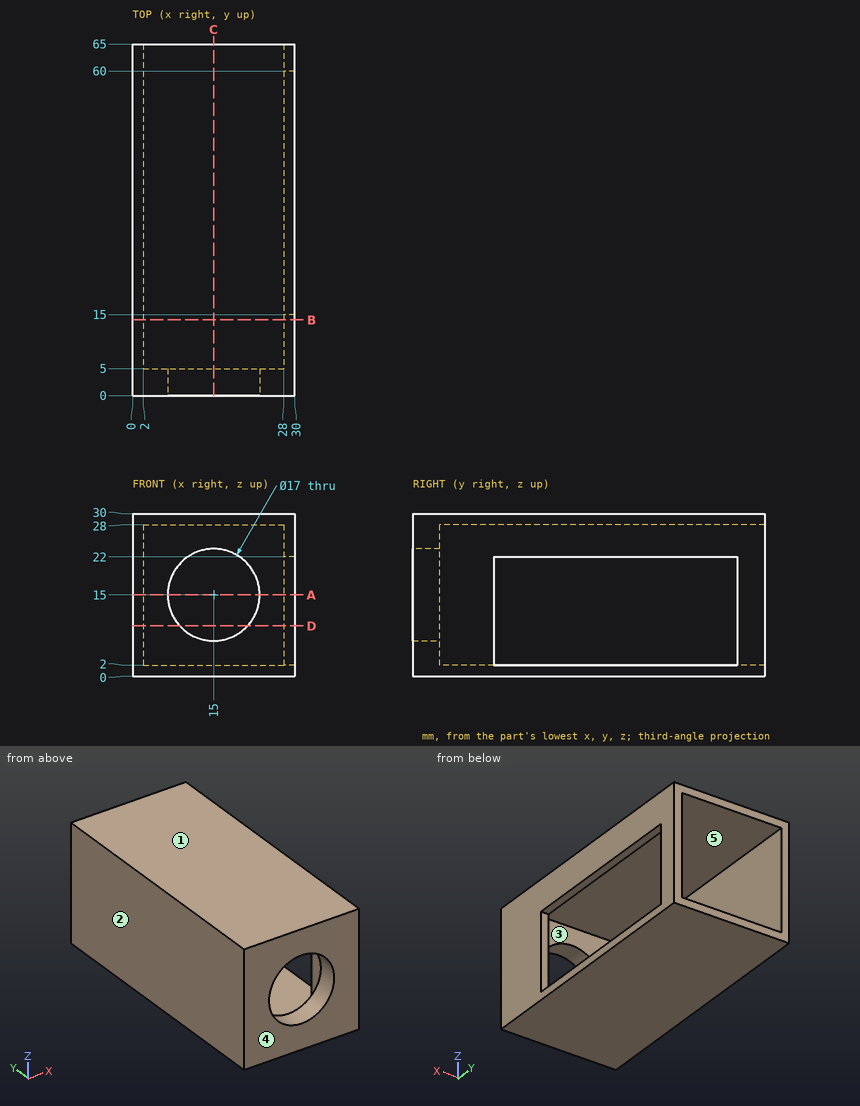
Design review of the part shown in the three views and the two pictorial views. Dimensions are in mm from the part's minimum x, y and z. A direction names the side the tool comes from. Give positions to 0.01 mm unless a question says otherwise; leave off trailing zeros. Loops run counter-clockwise (first coordinate to the right, second up) from the corner with the lowest first, then second, coordinate; pieces in that order, holes last. Notation, with made-up numbers: (79, -30) -> (91, -30) arc R9 cw to (91, -16) -> close; hole circle Ø1 at (-16.5, 74.25). An arc over 180 degrees is marked (long way). One line per question, with ' | ' between items.
1) We need section D-D (z = 9.25). Write out the cut boundary in (x, y).
Resolved:
outline: (0, 0) -> (8.74, 0) -> (8.74, 5) -> (2, 5) -> (2, 65) -> (0, 65) -> close; (21.26, 0) -> (30, 0) -> (30, 15) -> (28, 15) -> (28, 5) -> (21.26, 5) -> close; (28, 60) -> (30, 60) -> (30, 65) -> (28, 65) -> close
2) The part is to be moulded in two halves that separate along Z. For the marked faces 1, 2 and 3, say which applies: +Z half, -Z half, draft (parallel to the pull), parting line (faces both ways), or undercut.
Resolved:
face 1: +Z half | face 2: draft | face 3: undercut
3) To check wall thickness, follow probe 1 along X at (y, z) = (27, 26.25); probe 2 along X at (y, z) = (2.85, 15). State the ranges of each line that lie inside material, in increasing order.
Resolved:
probe 1: x = 0 to 2, 28 to 30 | probe 2: x = 0 to 6.5, 23.5 to 30
4) Insertion check: pin 1 Ø1.5 at (x, y) = (19, 54) entering from -Z; pin 2 Ø13 at (y, z) = (35.5, 10.5) entering from +X; pin 3 Ø12 at (x, z) = (13, 14) entering from -Y. Each pin has a flat end and moves straight along its axis. Give the tip position at first contact, or say it passes through.
Resolved:
pin 1: stops at z = 0 | pin 2: stops at x = 2 | pin 3: passes through
5) For the marked faces 4 and 5, list the 3-axis set-ups (+Z, -Z, +X, -X, +Y, -Y) from which the entire face can be reached by the end or side of a thin tool; tool diameter is ignored.
Resolved:
face 4: +Z, -Z, +X, -X, -Y | face 5: +Y
6) We need section A-A (z = 15). Write out the cut boundary in (x, y).
Resolved:
outline: (0, 0) -> (6.5, 0) -> (6.5, 5) -> (2, 5) -> (2, 65) -> (0, 65) -> close; (23.5, 0) -> (30, 0) -> (30, 15) -> (28, 15) -> (28, 5) -> (23.5, 5) -> close; (28, 60) -> (30, 60) -> (30, 65) -> (28, 65) -> close
7) We need section B-B (y = 14). Write out the cut boundary in (x, z).
Resolved:
outline: (0, 0) -> (30, 0) -> (30, 30) -> (0, 30) -> close; hole (2, 2) -> (28, 2) -> (28, 28) -> (2, 28) -> close
8) We need section C-C (x = 15). Write out the cut boundary in (y, z).
Resolved:
outline: (0, 0) -> (65, 0) -> (65, 2) -> (5, 2) -> (5, 6.5) -> (0, 6.5) -> close; (0, 23.5) -> (5, 23.5) -> (5, 28) -> (65, 28) -> (65, 30) -> (0, 30) -> close
